Geometry: see drawing. Coordinates: mm, zero at the bounding-box minimum. A direction names the side the tool comes from. Give positions to 0.01 mm unless a question says otherwise; leave off trailing zeros. Loops run counter-clockwise (first coordinate to the right, second up) from the corner with the lowest first, then second, coordinate; pieces in that order, holes last. Notation, with made-up numbers: (54.5, -39) -> (112.5, -39) arc R16 ccw to (112.5, -13) -> close; hole circle Ø10 at (-0.75, 86). An arc over 180 degrees is marked (long way). Return JSON: item names as keys, results as strings. Group by question number.
(1) Cut plane C-C on y = 20.5. Return loops of the section in (x, z).
(2) Cut plane A-A on z = 27.5. Return loops of the section in (x, y) (3 decimals), then the cut area to 3 significant figures.
(3) Cut plane B-B on x = 27.5. Return loops of the section in (y, z).
(4) Pin query (flat end, axial travel): pin 1 (3.5 mm diameter, centred on x = 27.5, y = 4, fed in from -Z); pin 2 (12 mm diameter, centred on y = 23.5, z = 16.5, fed in from +X); pin 3 (9 mm diameter, centred on x = 8.985, z = 27.5, fed in from -Y); pin 4 (4 mm diameter, centred on x = 27.5, z = 27.5, fed in from -Y). Return the tip coordinate at first contact, or that it passes through.
(5) Access query for the marked faces 1 and 2. Directions: +Z, -Z, +X, -X, +Y, -Y. A direction counts if a zero-diameter tool reaches every point of the face in a straight line with its end or side. Return the directions, or none.
(6) Draft query along X for the marked faces 3, 4 and 5. Return one class per face: released by +X, released by -X, zero draft, split by the parting line, or undercut.
(7) Ray query, line 1 (X direction, y = 26.75, z = 27.5) (3 decimals); line 2 (Y direction, x = 27.5, z = 23.55); line 3 (X direction, y = 5, z = 27.5). Return the intervals inside material, ascending. Write a range as from..to.
(8) Cut plane D-D on x = 45. Return loops of the section in (y, z).
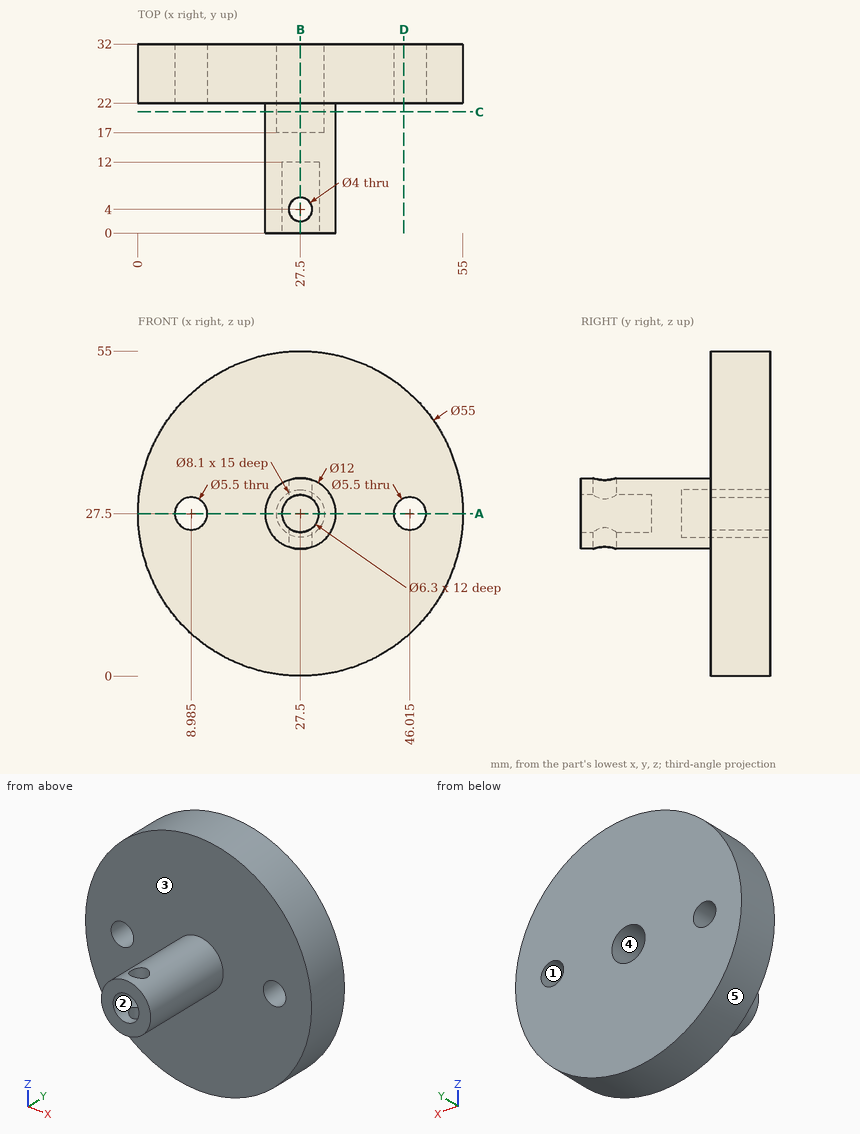
Answers:
{
 "1": {"outline": "circle Ø12 at (27.5, 27.5); hole circle Ø8.1 at (27.5, 27.5)"},
 "2": {"outline": "(0, 22) -> (6.235, 22) -> (6.235, 32) -> (0, 32) -> close; (11.735, 22) -> (21.5, 22) -> (21.5, 0) -> (24.35, 0) -> (24.35, 12) -> (30.65, 12) -> (30.65, 0) -> (33.5, 0) -> (33.5, 22) -> (43.265, 22) -> (43.265, 32) -> (31.55, 32) -> (31.55, 17) -> (23.45, 17) -> (23.45, 32) -> (11.735, 32) -> close; (48.765, 22) -> (55, 22) -> (55, 32) -> (48.765, 32) -> close", "area": "507 mm²"},
 "3": {"outline": "(0, 21.5) -> (2, 21.5) -> (2, 24.35) -> (0, 24.35) -> close; (0, 30.65) -> (2, 30.65) -> (2, 33.5) -> (0, 33.5) -> close; (6, 21.5) -> (22, 21.5) -> (22, 0) -> (32, 0) -> (32, 23.45) -> (17, 23.45) -> (17, 31.55) -> (32, 31.55) -> (32, 55) -> (22, 55) -> (22, 33.5) -> (6, 33.5) -> (6, 30.65) -> (12, 30.65) -> (12, 24.35) -> (6, 24.35) -> close"},
 "4": {"pin 1": "through", "pin 2": "x = 54.54", "pin 3": "y = 22", "pin 4": "y = 12"},
 "5": {"face 1": "+Y, -Y", "face 2": "-Y"},
 "6": {"face 3": "zero draft", "face 4": "undercut", "face 5": "split by the parting line"},
 "7": {"line 1": "0..6.235, 11.735..23.45, 31.55..43.265, 48.765..55", "line 2": "0..2, 6..17", "line 3": "21.5..24.35, 30.65..33.5"},
 "8": {"outline": "(22, 6.29) -> (32, 6.29) -> (32, 24.94) -> (22, 24.94) -> close; (22, 30.06) -> (32, 30.06) -> (32, 48.71) -> (22, 48.71) -> close"}
}
